from build123d import *

# Parameters (mm, degrees)
SKETCH_2_R          = 2
SKETCH_2_R_2        = 4
CUT_EXTRUDE_1_DEPTH = 36.860842154


with BuildPart() as part:
    # 草图1 → 旋转1 (revolve)
    with BuildSketch(Plane.XY, mode=Mode.PRIVATE) as revolve_1_sk:
        Polygon((0, 3), (-25, 3), (-25, 0), (-18.5, 0), (-18.5, -3), (0, -3), align=None)
    revolve(revolve_1_sk.sketch.rotate(Axis((0, 11.295290754, 0), (0, -1, 0)), 270), axis=Axis((0, 11.295290754, 0), (0, -1, 0)))

    # 草图2 → 切除-拉伸1 (cut, through all)
    with BuildSketch(Plane(origin=(0, 3, 0), x_dir=(1, 0, 0), z_dir=(0, 1, 0))):
        with Locations(Location((0, 15, 0), (0, 0, 270))):
            Circle(SKETCH_2_R)
        with Locations(Location((15, 0, 0), (0, 0, 270))):
            Circle(SKETCH_2_R)
        with Locations(Location((0, -15, 0), (0, 0, 270))):
            Circle(SKETCH_2_R)
        with Locations(Location((-15, 0, 0), (0, 0, 270))):
            Circle(SKETCH_2_R)
        with Locations(Location((0, 0, 0), (0, 0, 270))):
            Circle(SKETCH_2_R_2)
    extrude(amount=-CUT_EXTRUDE_1_DEPTH, mode=Mode.SUBTRACT)


solid = part.part
Can you work these out from the model? Positions are in its coordinate system, mm. Round coordinates to 2 decimals unless told otherwise and drop trailing zeros. Loops run counter-clockwise (first coordinate to the right, second up) from the corner with the lowest first, then second, coordinate; pieces in that order, holes last. Notation, with made-up numbers: (-2.5, 69.5) - (43.5, 69.5) arc R34 cw to (43.5, 102.5) - close; hole circle Ø6 at (69, 59.25). An arc over 180 degrees is marked (long way). Answer in a Markdown table with one row per item. Add a question column.
Q1. I want a section at C-C on x = -15. List the corners of the cut face in (y, z) for me, and give its area (3 significant figures).
Q2. For pin 1 Ø3 at (x, z) = (15, 0) entering from +Y; pin 2 Ø2 at (y, z) = (0, -14) entering from +X; pin 3 Ø1.5 at (x, y) = (11, 0) entering from +Z; pin 4 Ø2 at (x, y) = (13.5, 0.5) entering from -Z, each with a flat end and sliding along its axis, tell me the tip position at first contact or that it passes through.
Q3. I want a section at A-A on x = 0. List the corners of the cut face in (y, z) for me.
Q4. I want a section at B-B on z = 0. List the corners of the cut face in (x, y) for me.
Q5. I need wall thicknesses on L1, parallel to X at y = -1.1, z = 0; L2, parallel to X at y = 0.3, z = 0; L3, parallel to Z at x = 1, y = 2.7. Which ranges of each line are inside material? Lowest first, please.
Q6. We'd pull the mould along Z, two halves only. Please class faces 1 (the cylindrical face through (-3.905, 0.042, -0.867)), 2 (the cylindrical face through (7.086, -1.521, 17.089)), 3 (the cylindrical face through (-13, 0, 0)), 4 (the flat face through (-19, 0, 0)): pulls with the +Z half, pulls with the -Z half, needs draft (parallel to the pull), parting line crosses it, or undercut.
Q7. I want a section at D-D on y = 1.15. List the corners of the cut face in (x, z) for me.
A:
| question | item | result |
|---|---|---|
| 1 | outline | (-3, -10.83) - (0, -10.83) - (0, -20) - (3, -20) - (3, -2) - (-3, -2) - close; (-3, 2) - (3, 2) - (3, 20) - (0, 20) - (0, 10.83) - (-3, 10.83) - close |
| 1 | area | 161 mm^2 |
| 2 | pin 1 | through |
| 2 | pin 2 | x = 21.35 |
| 2 | pin 3 | z = 22.8 |
| 2 | pin 4 | z = -21.65 |
| 3 | outline | (-3, -18.5) - (0, -18.5) - (0, -25) - (3, -25) - (3, -17) - (-3, -17) - close; (-3, -13) - (3, -13) - (3, -4) - (-3, -4) - close; (-3, 4) - (3, 4) - (3, 13) - (-3, 13) - close; (-3, 17) - (3, 17) - (3, 25) - (0, 25) - (0, 18.5) - (-3, 18.5) - close |
| 4 | outline | (-25, 0) - (-18.5, 0) - (-18.5, -3) - (-17, -3) - (-17, 3) - (-25, 3) - close; (-13, -3) - (-4, -3) - (-4, 3) - (-13, 3) - close; (4, -3) - (13, -3) - (13, 3) - (4, 3) - close; (17, -3) - (18.5, -3) - (18.5, 0) - (25, 0) - (25, 3) - (17, 3) - close |
| 5 | L1 | -18.5 to -17, -13 to -4, 4 to 13, 17 to 18.5 |
| 5 | L2 | -25 to -17, -13 to -4, 4 to 13, 17 to 25 |
| 5 | L3 | -24.98 to -16.73, -13.27 to -3.87, 3.87 to 13.27, 16.73 to 24.98 |
| 6 | face 1 | undercut |
| 6 | face 2 | parting line crosses it |
| 6 | face 3 | undercut |
| 6 | face 4 | needs draft |
| 7 | outline | circle Ø50 at (0, 0); hole circle Ø4 at (-15, 0); hole circle Ø8 at (0, 0); hole circle Ø4 at (0, -15); hole circle Ø4 at (0, 15); hole circle Ø4 at (15, 0) |
